Design review of the part built by this model. Coordinates are the model's own, in mm. Face numbers are marked on the shaded views. A direction names the side the tool comes from. Give positions to 0.01 mm unless a question says otherwise; leave off trailing zeros. Order: outer loops, then holes, each group sorted by start corner. A loop starts at its lowest first (then second) coordinate and runs counter-clockwise, first axis right, second up. Notation, with made-up numbers: (22, -25.75) -> (27, -25.75) arc R14 cw to (27, -1.75) -> close; hole circle Ø4 at (20, -14). An arc over 180 degrees is marked (long way). One line per item, written item: value. Start each with the question number.
1) Wall thickness on line 1 along X through (y, z) = (4.1, 6.5); line 2 along X through (y, z) = (1.35, 6.5); line 3 along Y through (x, z) = (28, 3): over which ranges is each line inside the solid? List them lowest first. Write a range as from..to.
2) Consider section C-C (z = 2.25). State the section outline as (x, y) points.
3) For pin 1 (5 mm diameter, centred on x = 21.5, z = 1.5, fed in from -Y); pin 2 (3 mm diameter, centred on x = 19, z = 5.5, fed in from +Y); pin 3 (3 mm diameter, centred on x = 26, z = 8, fed in from -Y); pin 4 (1.4 mm diameter, centred on x = 25.5, z = 4, fed in from +Y), all flat-tipped, find the tip position at first contact; note any pin that passes through.
4) Consider section B-B (z = 6.5). State the section outline as (x, y) points, plus the area to 3 significant figures.
5) Tool access review of the marked faces 1 and 2: name each direction out of +Z, -Z, +X, -X, +Y, -Y from which nothing blocks a thin tool from reaching the whole face with its end or side.
6) Consider section A-A (x = 32). State the section outline as (y, z) points.
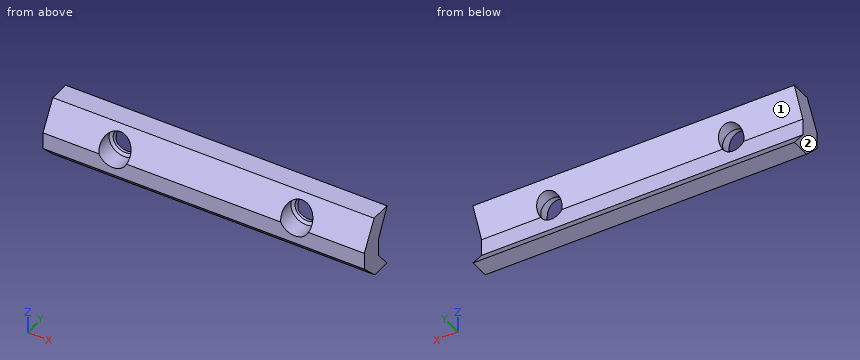
from build123d import *

# Parameters (mm, degrees)
F1_DEPTH = 53
F3_D     = 4
F3_DEPTH = 7.5
F3_START = 1.7320508
F3_TIP   = 1.2017212381
F4_D     = 4
F4_DEPTH = 7.5
F4_START = 1.7320508
F4_TIP   = 1.2017212381
F5_D     = 5
F5_DEPTH = 1
F5_START = 2.0207259
F5_TIP   = 1.5021515476
F6_D     = 5
F6_DEPTH = 1
F6_START = 2.0207259
F6_TIP   = 1.5021515476


with BuildPart() as f1:
    # F0 (on Right) → F1 (new body)
    with BuildSketch(Plane.YZ):
        Polygon((0, 2.75), (2.75, 0), (6, 0), (3.75, 2.75), (3.75, 5.5), (6, 10), (2.5980762114, 10), (0, 5.5), align=None)
    extrude(amount=F1_DEPTH)

    # F3
    # its depths count from where the whole tool has entered the part; down to there all is cleared
    with Locations(Plane.XZ.offset(-F3_START)):
        with Locations((11.5, 6.5)):
            Hole(F3_D / 2, depth=F3_DEPTH)
            with Locations((0, 0, -(F3_DEPTH + F3_TIP / 2))):  # 118° drill point
                Cone(0, F3_D / 2, F3_TIP, mode=Mode.SUBTRACT)

    # F4
    # its depths count from where the whole tool has entered the part; down to there all is cleared
    with Locations(Plane.XZ.offset(-F4_START)):
        with Locations((41.5, 6.5)):
            Hole(F4_D / 2, depth=F4_DEPTH)
            with Locations((0, 0, -(F4_DEPTH + F4_TIP / 2))):  # 118° drill point
                Cone(0, F4_D / 2, F4_TIP, mode=Mode.SUBTRACT)

    # F5
    # its depths count from where the whole tool has entered the part; down to there all is cleared
    with Locations(Plane.XZ):
        with Locations((11.5, 6.5)):
            Hole(F5_D / 2, depth=F5_START)
    with Locations(Plane.XZ.offset(-F5_START)):
        with Locations((11.5, 6.5)):
            Hole(F5_D / 2, depth=F5_DEPTH)
            with Locations((0, 0, -(F5_DEPTH + F5_TIP / 2))):  # 118° drill point
                Cone(0, F5_D / 2, F5_TIP, mode=Mode.SUBTRACT)

    # F6
    # its depths count from where the whole tool has entered the part; down to there all is cleared
    with Locations(Plane.XZ):
        with Locations((41.5, 6.5)):
            Hole(F6_D / 2, depth=F6_START)
    with Locations(Plane.XZ.offset(-F6_START)):
        with Locations((41.5, 6.5)):
            Hole(F6_D / 2, depth=F6_DEPTH)
            with Locations((0, 0, -(F6_DEPTH + F6_TIP / 2))):  # 118° drill point
                Cone(0, F6_D / 2, F6_TIP, mode=Mode.SUBTRACT)


solid = f1.part
Checked values:
1. line 1: x = 0..9.5, 13.5..39.5, 43.5..53
1. line 2: x = 0..9, 14..39, 44..53
1. line 3: y = 0..3.75
2. outline: (0, 0.5) -> (53, 0.5) -> (53, 4.16) -> (0, 4.16) -> close
3. pin 1: stops at y = 0
3. pin 2: stops at y = 4.5
3. pin 3: stops at y = 0.58
3. pin 4: stops at y = 3.75
4. outline: (0, 0.58) -> (9, 0.58) -> (9, 3.02) -> (9.5, 3.32) -> (9.5, 4.25) -> (0, 4.25) -> close; (13.5, 3.32) -> (14, 3.02) -> (14, 0.58) -> (39, 0.58) -> (39, 3.02) -> (39.5, 3.32) -> (39.5, 4.25) -> (13.5, 4.25) -> close; (43.5, 3.32) -> (44, 3.02) -> (44, 0.58) -> (53, 0.58) -> (53, 4.25) -> (43.5, 4.25) -> close
4. area: 160 mm^2
5. face 1: +X, -X, +Y
5. face 2: +Z, -Z, -X, +Y, -Y
6. outline: (0, 2.75) -> (2.75, 0) -> (6, 0) -> (3.75, 2.75) -> (3.75, 5.5) -> (6, 10) -> (2.6, 10) -> (0, 5.5) -> close
